Here's how the part is built. I have some questions about the finished solid (model axes, mm). Coordinates: 2 decimals unless noted, no trailing zeros. Write each loop counter-clockwise with the first axis right and the second up, starting at its lowest first coordinate (ties: lowest second). Pieces come first, ordered by that corner, then holes.
Item 1: If we section it at C-C (y = 23): Please give me the cut outline in (x, z).
Item 2: I'm going to push a flat-ended pin straight in: pin 1 Ø12 at (x, y) = (1, -12.5) entering from +Z. Where does the tip first touch, or does it pass through?
Item 3: If we section it at D-D (x = -2.25): Please give me the cut outline in (y, z), then the cut area to 3 significant figures.
Item 4: If I drill on line 1 (Y direction, x = 2.25, z = 0.6); line 2 (X direction, y = 12.5, z = 1.15); line 3 (Y direction, x = 2.5, z = 1.2), over which ranges is the centre line in solid material (lowest first)?
Item 5: If we section it at A-A (x = 3.25): Please give me the cut outline in (y, z).
Item 6: If we section it at B-B (z = 0.55): Please give me the cut outline in (x, y).
from build123d import *

# Parameters (mm, degrees)
SKETCH1_R            = 2
BOSS_EXTRUDE1_DEPTH  = 1.5875
FILLET2_R            = 1.778
M4_CLEARANCE_HOLE2_D = 4.5


with BuildPart() as part:
    # Sketch1 → Boss-Extrude1 (new body)
    with BuildSketch(Plane.XY):
        with BuildLine():
            Line((-3.078924099, -28.617866551), (2.159951047, -28.617866551))
            Line((2.159951047, -28.617866551), (7.398508015, -28.617866551))
            Line((7.398508015, -28.617866551), (7.398508015, 29.568125765))
            Line((7.398508015, 29.568125765), (13.896694252, 66.719401178))
            ThreePointArc((13.896694252, 66.719401178), (2.158041982, 59.568125704), (-9.580610288, 66.719401178))
            Line((-9.580610288, 66.719401178), (-3.078924099, 29.568125765))
            Line((-3.078924099, 29.568125765), (-3.078924099, -28.617866551))
        make_face()
        with BuildLine():
            ThreePointArc((4.159951047, -14.006866551), (3.574164609, -15.421080114), (2.159951047, -16.006866551))
            ThreePointArc((2.159951047, -16.006866551), (0.745737485, -12.592652989), (4.159951047, -14.006866551))
        make_face(mode=Mode.SUBTRACT)
        with Locations((2.159951047, 14.957125769)):
            Circle(SKETCH1_R, mode=Mode.SUBTRACT)
    extrude(amount=BOSS_EXTRUDE1_DEPTH)

    # Fillet2
    fillet2_edges = [part.edges().sort_by_distance(p)[0] for p in [
        (-9.580610288, 66.719401178, 0.79375),
        (13.896694252, 66.719401178, 0.79375),
        (7.398508015, -28.617866551, 0.79375),
        (-3.078924099, -28.617866551, 0.79375),
    ]]
    fillet(fillet2_edges, radius=FILLET2_R)

    # M4 Clearance Hole2 (through all)
    with Locations(Plane.XY.offset(1.5875)):
        with Locations((2.159951047, 14.957125769), (2.159951047, -14.006866551)):
            Hole(M4_CLEARANCE_HOLE2_D / 2)


solid = part.part
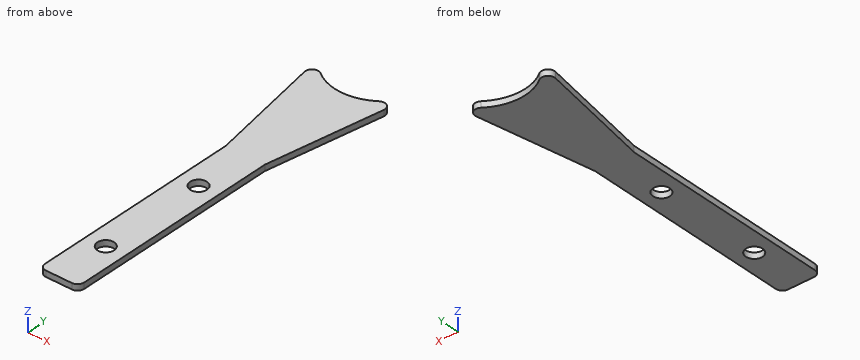
Answer list:
1. outline: (-3.08, 0) - (7.4, 0) - (7.4, 1.59) - (-3.08, 1.59) - close
2. pin 1: stops at z = 1.59
3. outline: (-28.34, 0) - (60.33, 0) - (60.33, 1.59) - (-28.34, 1.59) - close
3. area: 141 mm2
4. line 1: y = -28.62 to -16.26, -11.76 to 12.71, 17.21 to 59.57
4. line 2: x = -3.08 to 7.4
4. line 3: y = -28.62 to -16.23, -11.78 to 12.73, 17.18 to 59.57
5. outline: (-28.62, 0) - (-15.98, 0) - (-15.98, 1.59) - (-28.62, 1.59) - close; (-12.04, 0) - (12.99, 0) - (12.99, 1.59) - (-12.04, 1.59) - close; (16.93, 0) - (59.61, 0) - (59.61, 1.59) - (16.93, 1.59) - close
6. outline: (-8.47, 60.4) - (-3.08, 29.57) - (-3.08, -26.84) arc R1.78 ccw to (-1.3, -28.62) - (5.62, -28.62) arc R1.78 ccw to (7.4, -26.84) - (7.4, 29.57) - (12.79, 60.4) arc R1.78 ccw to (9.99, 62.14) arc R13.21 cw to (-5.67, 62.14) arc R1.78 ccw to start; hole circle Ø4.5 at (2.16, -14.01); hole circle Ø4.5 at (2.16, 14.96)
